Design review of the part built by this model. Coordinates are the model's own, in mm. Round coordinates to 2 decimals unless told otherwise and drop trailing zeros. Loops run counter-clockwise (first coordinate to the right, second up) from the corner with the lowest first, then second, coordinate; pieces in that order, holes last. Notation, with made-up numbers: (-1.5, -31.5) - (19.5, -31.5) arc R22 cw to (19.5, 1.5) - close; hole circle Ø10 at (52, 51.25). An arc over 180 degrees is marked (long way). Use one line per item in the form item = value. Start each with the question number.
(1) We need section B-B, the plane x = -147. Write out the cut boundary in (y, z), then the cut area to 3 significant figures.
(2) Wall thickness on probe 1 along Y at (x, z) = (-107.5, 67.5); probe 2 along Y at (x, z) = (-155, 68); probe 3 along X at (y, z) = (-31, 67.6): over which ranges is each line inside the solid? List them lowest first. Write a range as [from, to].
(3) The part is to be moulded in two halves that separate along X. For faces 1 (the flat face through (-125, 1, 66.5)), 2 (the flat face through (-158, -1, 68)), 3 (the cylindrical face through (-149.88, -11.99, 67.77)), 4 (the cylindrical face through (-104.7, 33.07, 67.77)), say which applies: released by +X, released by -X, zero draft, split by the parting line, or undercut.
(4) We need section C-C, the plane y = 22.5. Write out the cut boundary in (x, z), then the cut area to 3 significant figures.
(5) We need section D-D, the plane z = 68.05. Give the number of separate pieces and of enclosed holes in the cut face, then the cut area to 3 significant figures.
(6) For pin 1 (2 mm diameter, centred on x = -116.5, y = -12.5, fed in from -Z), flat-tipped, find the tip position at first contact; note if it passes through.
(7) We need section A-A, the plane y = -30.5. Write out the cut boundary in (x, z).
from build123d import *

# Parameters (mm, degrees)
MAIN_PROFILE_SKETCH_R = 1.7
MAIN_EXTRUSION_DEPTH  = 2.5


with BuildPart() as part:
    # Main Profile Sketch → Main Extrusion (new body)
    with BuildSketch(Plane.XY.offset(69)):
        with BuildLine():
            Line((-158, 53), (-93.05122926, 53))
            ThreePointArc((-93.05122926, 53), (-93.300513342, 50.683537094), (-92, 48.750454583))
            Line((-92, 48.750454583), (-92, -48.750454583))
            ThreePointArc((-92, -48.750454583), (-93.300513342, -50.683537094), (-93.05122926, -53))
            Line((-93.05122926, -53), (-158, -53))
            Line((-158, -53), (-158, 53))
        make_face()
        with Locations((-155, -45)):
            Circle(MAIN_PROFILE_SKETCH_R, mode=Mode.SUBTRACT)
        with Locations((-142.5, -47.5)):
            Circle(MAIN_PROFILE_SKETCH_R, mode=Mode.SUBTRACT)
        with Locations((-142.5, -30.5)):
            Circle(MAIN_PROFILE_SKETCH_R, mode=Mode.SUBTRACT)
        with Locations((-151.5, -12.5)):
            Circle(MAIN_PROFILE_SKETCH_R, mode=Mode.SUBTRACT)
        with Locations((-133.5, -12.5)):
            Circle(MAIN_PROFILE_SKETCH_R, mode=Mode.SUBTRACT)
        with Locations((-107.5, -47.5)):
            Circle(MAIN_PROFILE_SKETCH_R, mode=Mode.SUBTRACT)
        with Locations((-95, -45)):
            Circle(MAIN_PROFILE_SKETCH_R, mode=Mode.SUBTRACT)
        with Locations((-107.5, -30.5)):
            Circle(MAIN_PROFILE_SKETCH_R, mode=Mode.SUBTRACT)
        with Locations((-116.5, -12.5)):
            Circle(MAIN_PROFILE_SKETCH_R, mode=Mode.SUBTRACT)
        with Locations((-98.5, -12.5)):
            Circle(MAIN_PROFILE_SKETCH_R, mode=Mode.SUBTRACT)
        with Locations((-151.5, 22.5)):
            Circle(MAIN_PROFILE_SKETCH_R, mode=Mode.SUBTRACT)
        with Locations((-133.5, 22.5)):
            Circle(MAIN_PROFILE_SKETCH_R, mode=Mode.SUBTRACT)
        with Locations((-147, 33)):
            Circle(MAIN_PROFILE_SKETCH_R, mode=Mode.SUBTRACT)
        with Locations((-155, 45)):
            Circle(MAIN_PROFILE_SKETCH_R, mode=Mode.SUBTRACT)
        with Locations((-147, 47)):
            Circle(MAIN_PROFILE_SKETCH_R, mode=Mode.SUBTRACT)
        with Locations((-116.5, 22.5)):
            Circle(MAIN_PROFILE_SKETCH_R, mode=Mode.SUBTRACT)
        with Locations((-98.5, 22.5)):
            Circle(MAIN_PROFILE_SKETCH_R, mode=Mode.SUBTRACT)
        with Locations((-103, 33)):
            Circle(MAIN_PROFILE_SKETCH_R, mode=Mode.SUBTRACT)
        with Locations((-103, 47)):
            Circle(MAIN_PROFILE_SKETCH_R, mode=Mode.SUBTRACT)
        with Locations((-95, 45)):
            Circle(MAIN_PROFILE_SKETCH_R, mode=Mode.SUBTRACT)
    extrude(amount=-MAIN_EXTRUSION_DEPTH)


solid = part.part
Data:
q1.outline = (-53, 66.5) - (31.3, 66.5) - (31.3, 69) - (-53, 69) - close; (34.7, 66.5) - (45.3, 66.5) - (45.3, 69) - (34.7, 69) - close; (48.7, 66.5) - (53, 66.5) - (53, 69) - (48.7, 69) - close
q1.area = 248 mm^2
q2.probe_1 = [-53, -49.2], [-45.8, -32.2], [-28.8, 53]
q2.probe_2 = [-53, -46.7], [-43.3, 43.3], [46.7, 53]
q2.probe_3 = [-158, -144.12], [-140.88, -109.12], [-105.88, -92]
q3.face_1 = zero draft
q3.face_2 = released by -X
q3.face_3 = undercut
q3.face_4 = undercut
q4.outline = (-158, 66.5) - (-153.2, 66.5) - (-153.2, 69) - (-158, 69) - close; (-149.8, 66.5) - (-135.2, 66.5) - (-135.2, 69) - (-149.8, 69) - close; (-131.8, 66.5) - (-118.2, 66.5) - (-118.2, 69) - (-131.8, 69) - close; (-114.8, 66.5) - (-100.2, 66.5) - (-100.2, 69) - (-114.8, 69) - close; (-96.8, 66.5) - (-92, 66.5) - (-92, 69) - (-96.8, 69) - close
q4.area = 131 mm^2
q5.separate_pieces = 1
q5.enclosed_holes = 20
q5.area = 6,810 mm^2
q6.pin_1 = through
q7.outline = (-158, 66.5) - (-144.2, 66.5) - (-144.2, 69) - (-158, 69) - close; (-140.8, 66.5) - (-109.2, 66.5) - (-109.2, 69) - (-140.8, 69) - close; (-105.8, 66.5) - (-92, 66.5) - (-92, 69) - (-105.8, 69) - close
